For this review, use the dimensioned drawing (mm, ordinates from the lowest corner) and the shaded views. Give positions to 0.01 mm unless a question says otherwise; leave off trailing zeros. Order: outer loops, then holes, each group sorted by start corner. A loop starts at its lowest first (then second) coordinate and runs counter-clockwise, first axis right, second up.
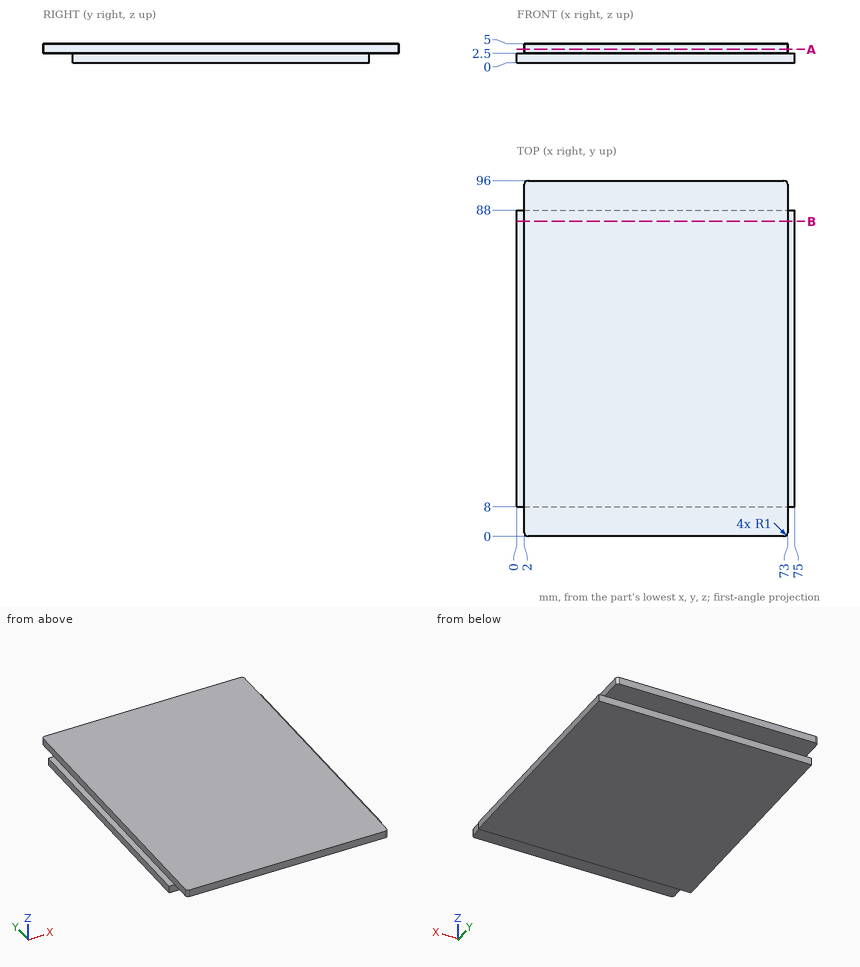
1. For pin 1 (6.5 mm diameter, centred on x = 35, y = 3.5, fed in from -Z); pin 2 (6 mm diameter, centred on x = 23, y = 43, fed in from -Z); pin 3 (1 mm diameter, centred on x = 1, y = 33.5, fed in from +Z); pin 4 (0.8 mm diameter, centred on y = 44, z = 3, fed in from -X), all flat-tipped, find the tip position at first contact; note any pin that passes through.
Recorded:
pin 1: stops at z = 2.5
pin 2: stops at z = 0
pin 3: stops at z = 2.5
pin 4: stops at x = 2
2. Take a section at A-A (z = 3.55). State the section outline as (x, y) points.
Recorded:
outline: (2, 1) arc R1 ccw to (3, 0) - (72, 0) arc R1 ccw to (73, 1) - (73, 95) arc R1 ccw to (72, 96) - (3, 96) arc R1 ccw to (2, 95) - close
3. For line 1 along X through (y, z) = (13, 4.25); line 2 along Z through (x, y) = (8, 4.5); line 3 along Y through (x, z) = (69, 0.8), list the stretches that pass through material, from the lowest coordinate up.
Recorded:
line 1: x = 2 to 73
line 2: z = 2.5 to 5
line 3: y = 8 to 88
4. Take a section at B-B (y = 85). State the section outline as (x, z) points, then the cut area to 3 significant figures.
Recorded:
outline: (0, 0) - (75, 0) - (75, 2.5) - (73, 2.5) - (73, 5) - (2, 5) - (2, 2.5) - (0, 2.5) - close
area: 365 mm2
